from build123d import *

# Parameters (mm, degrees)
SKETCH_1_R          = 9
EXTRUDE_1_DEPTH     = 40
SKETCH_2_R          = 3.2
CUT_EXTRUDE_1_DEPTH = 17
SKETCH_15_W         = 8.3
SKETCH_15_H         = 8.3
EXTRUDE_2_DEPTH     = 10
SKETCH_16_R         = 4.2
CUT_EXTRUDE_2_DEPTH = 10
SKETCH_17_R         = 1.6
CUT_EXTRUDE_3_DEPTH = 10


with BuildPart() as part:
    # 草图1 → 凸台-拉伸1 (new body)
    with BuildSketch(Plane(origin=(0, 0, 0), x_dir=(1, 0, 0), z_dir=(0, 1, 0))):
        Circle(SKETCH_1_R)
    extrude(amount=EXTRUDE_1_DEPTH)

    # 草图2 → 切除-拉伸1 (cut)
    with BuildSketch(Plane.XZ):
        Circle(SKETCH_2_R)
    extrude(amount=-CUT_EXTRUDE_1_DEPTH, mode=Mode.SUBTRACT)

    # 草图15 → 凸台-拉伸2 (add)
    with BuildSketch(Plane(origin=(0, 40, 0), x_dir=(1, 0, 0), z_dir=(0, 1, 0))):
        Rectangle(SKETCH_15_W, SKETCH_15_H)
    extrude(amount=EXTRUDE_2_DEPTH)

    # 草图16 → 切除-拉伸2 (cut, symmetric)
    with BuildSketch(Plane.XY):
        with Locations((0, 22)):
            Circle(SKETCH_16_R)
    extrude(amount=CUT_EXTRUDE_2_DEPTH, both=True, mode=Mode.SUBTRACT)

    # 草图17 → 切除-拉伸3 (cut, symmetric)
    with BuildSketch(Plane(origin=(0, 0, 0), x_dir=(0, 0, -1), z_dir=(1, 0, 0))):
        with Locations((0, 22)):
            Circle(SKETCH_17_R)
    extrude(amount=CUT_EXTRUDE_3_DEPTH, both=True, mode=Mode.SUBTRACT)


solid = part.part
Source: CAD feature listing. Evaluate the final solid. Frame: model axes, mm. A direction names the side the tool comes from. Round coordinates to 2 decimals unless told otherwise and drop trailing zeros. Loops run counter-clockwise (first coordinate to the right, second up) from the corner with the lowest first, then second, coordinate; pieces in that order, holes last. Notation, with made-up numbers: M 7,68.25 L 30,68.25 A21 cw 30,91.25 Z; hole C -36.75,3 d1. An arc over 180 degrees is marked long. Answer as CSV lines item,"result".
Q1. Pull-direction query (Y, two-part tool) for faces 5 (the face through (-4.15, 45, 0)), 6 (the face through (-6.41, 22.07, 1.6)), 7 (the face through (0, 0, 4)); classes: +Y half, -Y half, draft (parallel to the pull), parting line (faces both ways), or undercut.
Verdict:
face 5,"draft"
face 6,"undercut"
face 7,"-Y half"
Q2. Reachability of faces 1 (the face through (-2.539, 8.381, -1.947)), 2 (the face through (0, 45, -4.15)), 3 (the face through (0, 45, 4.15)), 4 (the face through (4.15, 45, 0)) from +Z, -Z, +X, -X, +Y, -Y: full face, straight path, thin tool, end or side. Return the list, or none.
Verdict:
face 1,"-Y"
face 2,"-Z, +X, -X, +Y"
face 3,"+Z, +X, -X, +Y"
face 4,"+Z, -Z, +X, +Y"
Q3. Cut plane C-C (y = 22). Return the cut outline in (x, z), plus the area to 3 significant figures.
Verdict:
outline,"M -8.86,-1.6 A9 ccw -4.2,-7.96 L -4.2,-1.6 Z; M -8.86,1.6 L -4.2,1.6 L -4.2,7.96 A9 ccw Z; M 4.2,-7.96 A9 ccw 8.86,-1.6 L 4.2,-1.6 Z; M 4.2,1.6 L 8.86,1.6 A9 ccw 4.2,7.96 Z"
area,"78.5 mm^2"
Q4. Contact query for flat-ended pins moving along their axis: pin 1 (6.5 mm diameter, centred on x = -0.5, y = 43, fed in from +Z); pin 2 (3 mm diameter, centred on x = 1.5, y = 44, fed in from -Z); pin 3 (6.5 mm diameter, centred on y = 45.5, z = -2, fed in from -X); pin 4 (6.5 mm diameter, centred on y = 46.5, z = 1, fed in from +X). Output: stop coordinate, or through.
Verdict:
pin 1,"stops at z = 9"
pin 2,"stops at z = -4.15"
pin 3,"stops at x = -4.15"
pin 4,"stops at x = 4.15"
Q5. Cut plane D-D (y = 15). Return the cut outline in (x, z).
Verdict:
outline,"C 0,0 d18; hole C 0,0 d6.4"
Q6. Line query: line 1 along Z through (x, y) = (0, 7); line 2 along Y through (x, z) = (6.15, 0); line 3 along Y through (x, z) = (0, -3.5). Output: solid intervals per line, ascending.
Verdict:
line 1,"z = -9 to -3.2, 3.2 to 9"
line 2,"y = 0 to 20.4, 23.6 to 40"
line 3,"y = 0 to 17.8, 26.2 to 50"
Q7. Cut plane A-A (x = 0). Return the cut outline in (y, z), plus the area to 3 significant figures.
Verdict:
outline,"M 0,-9 L 17.8,-9 L 17.8,9 L 0,9 L 0,3.2 L 17,3.2 L 17,-3.2 L 0,-3.2 Z; M 26.2,-9 L 40,-9 L 40,-4.15 L 50,-4.15 L 50,4.15 L 40,4.15 L 40,9 L 26.2,9 Z"
area,"543 mm^2"
Q8. Cut plane B-B (z = 0). Return the cut outline in (x, y).
Verdict:
outline,"M -9,0 L -3.2,0 L -3.2,17 L 3.2,17 L 3.2,0 L 9,0 L 9,20.4 L 3.88,20.4 A4.2 cw -3.88,20.4 L -9,20.4 Z; M -9,23.6 L -3.88,23.6 A4.2 cw 3.88,23.6 L 9,23.6 L 9,40 L 4.15,40 L 4.15,50 L -4.15,50 L -4.15,40 L -9,40 Z"
